Part model, mm, in its own coordinate system. Face numbers are marked on the shaded views. A direction names the side the tool comes from. Give positions to 0.01 mm unless a question says otherwise; leave off trailing zeros. Order: outer loops, then holes, each group sorted by start corner. A loop starts at its lowest first (then second) coordinate and runs counter-clockwise, first axis right, second up. Notation, with made-up numbers: M 27.5,74.5 L 47.5,74.5 A6 ccw 47.5,81.5 Z; hole C -30.5,78.5 d6. An arc over 180 degrees is marked long. Return JSON: item names as keys, results as strings.
Autodesk Inventor part; units mm, degrees
ref_plane "YZ Plane" through (0, 0, 0) normal (1, 0, 0) x (0, 1, 0)
ref_plane "XZ Plane" through (0, 0, 0) normal (0, 1, 0) x (-1, 0, 0)
ref_plane "XY Plane" through (0, 0, 0) normal (0, 0, 1) x (1, 0, 0)
sketch "Sketch1" plane through (0, 0, 0) normal (0, 1, 0) x (-1, 0, 0)
  line L0 (7.5, 7.5) -> (-7.5, 7.5)
  line L1 (-7.5, 7.5) -> (-7.5, -7.5)
  line L2 (-7.5, -7.5) -> (7.5, -7.5)
  line L3 (7.5, -7.5) -> (7.5, 7.5)
  line L4 (7.5, 7.5) -> (-7.5, -7.5) construction
  line L5 (-7.5, 7.5) -> (7.5, -7.5) construction
  line L6 (7.5, 7.5) -> (5.5, 7.5)
  line L7 (5.5, 7.5) -> (5.5, -7.5)
  line L8 (5.5, -7.5) -> (7.5, -7.5)
  line L9 (7.5, -7.5) -> (7.5, 7.5)
  circle A0 centre (0, 3) radius 1.5
  circle A1 centre (0, 3) radius 2.75
  line L10 (7.5, 0) -> (-7.5, 0) construction
  line L11 (0, 7.5) -> (0, -7.5) construction
  circle A2 centre (0, -3) radius 1.5
  circle A3 centre (0, -3) radius 2.75
  point P0 (0, 0)
  dimension "d0" = 15
  dimension "d1" = 15
  dimension "d2" = 2
  dimension "d3" = 3
  dimension "d4" = 5.5
  dimension "d5" = 4.5
extrude "Extrusion1" add sketch "Sketch1" along normal blind 2 contours L7 L2 L1 L0
extrude "Extrusion2" add sketch "Sketch1" along normal blind 1 contours A1 | A3
extrude "Extrusion3" add sketch "Sketch1" along normal blind 28 contours L3 L2 L7 L0
sketch "Sketch2" plane through (-5.5, 2, -7.5) normal (1, 0, 0) x (0, 0, -1)
  circle A0 centre (-7.5, 8.5) radius 1.5
  line L0 (-15, 0) -> (0, 0)
  circle A1 centre (-7.5, 20.5) radius 1.5
  point P0 (-7.5, -2)
  dimension "d12" = 3
  dimension "d13" = 8.5
  dimension "d14" = 3
  dimension "d15" = 20.5
extrude "Extrusion4" cut sketch "Sketch2" against normal blind 2
properties part number "Konektor Lifter 2_3DPrint"
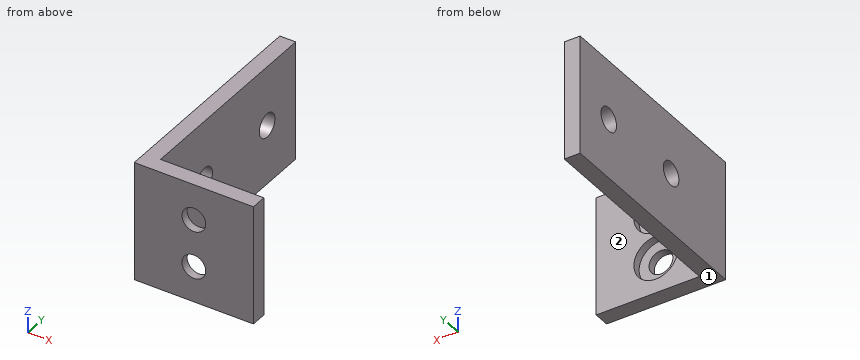
Q1. Band-saw the part on A-A (y = 22.5). Give the cut face in (x, z).
Established:
{"outline": "M -7.5,-7.5 L -5.5,-7.5 L -5.5,-1.5 L -7.5,-1.5 Z; M -7.5,1.5 L -5.5,1.5 L -5.5,7.5 L -7.5,7.5 Z"}
Q2. Band-saw the part on D-D (z = -2.5). Give the cut face in (x, y).
Established:
{"outline": "M -7.5,0 L -1.41,0 L -1.41,1 L -2.7,1 L -2.7,2 L -5.5,2 L -5.5,28 L -7.5,28 Z; M 1.41,0 L 7.5,0 L 7.5,2 L 2.7,2 L 2.7,1 L 1.41,1 Z"}
Q3. 3-axis set-ups, long thin cutter, end or side, ignore diameter. For the marked faces 1 and 2: which of +Z, -Z, +X, -X, +Y, -Y reach the whole face in a straight line?
Established:
{"face 1": "-Z, +X, -X, +Y, -Y", "face 2": "+Z, -Z, +X, +Y"}
Q4. Band-saw the part on B-B (z = 3). Give the cut face in (x, y).
Established:
{"outline": "M -7.5,0 L -1.5,0 L -1.5,1 L -2.75,1 L -2.75,2 L -5.5,2 L -5.5,28 L -7.5,28 Z; M 1.5,0 L 7.5,0 L 7.5,2 L 2.75,2 L 2.75,1 L 1.5,1 Z"}
Q5. Band-saw the part on C-C (x = 0). Give the cut face in (y, z).
Established:
{"outline": "M 0,-7.5 L 2,-7.5 L 2,-5.75 L 1,-5.75 L 1,-4.5 L 0,-4.5 Z; M 0,-1.5 L 1,-1.5 L 1,-0.25 L 2,-0.25 L 2,0.25 L 1,0.25 L 1,1.5 L 0,1.5 Z; M 0,4.5 L 1,4.5 L 1,5.75 L 2,5.75 L 2,7.5 L 0,7.5 Z"}
Q6. Probe line 1 along Z through (x, y) = (0, 1.75); line 2 along Z through (x, y) = (0, 0.4); line 3 along Y through (x, z) = (0.25, 1.25). List the from-to ranges inside material, lowest first.
Established:
{"line 1": "z = -7.5 to -5.75, -0.25 to 0.25, 5.75 to 7.5", "line 2": "z = -7.5 to -4.5, -1.5 to 1.5, 4.5 to 7.5", "line 3": "y = 0 to 1"}
Q7. Pin check, flat tips, straight feed: pin 1 (2 mm diameter, centred on x = -3.5, z = -0.5, fed in from +Y); pin 2 (4 mm diameter, centred on y = 22.5, z = 0, fed in from +X). Stop position of each tip, or through.
Established:
{"pin 1": "stops at y = 2", "pin 2": "stops at x = -5.5"}
